```python
from build123d import *

# Parameters (mm, degrees)
SKETCH1_W               = 100
SKETCH1_H               = 100
BOSS_EXTRUDE1_DEPTH     = 20
SKETCH3_R               = 7.1
CUT_EXTRUDE1_DEPTH      = 16.5
CUT_EXTRUDE4_DEPTH      = 74.484692283
CUT_EXTRUDE4_DEPTH_BACK = 74.484692283
SKETCH7_R               = 6.1
FILLET1_R               = 3
SKETCH11_W              = 24
SKETCH11_H              = 24
CUT_EXTRUDE6_DEPTH      = 15
SKETCH12_W              = 18
SKETCH12_H              = 15
CUT_EXTRUDE7_DEPTH      = 32


with BuildPart() as part:
    # Sketch1 → Boss-Extrude1 (new body)
    with BuildSketch(Plane(origin=(0, 0, 0), x_dir=(1, 0, 0), z_dir=(0, 1, 0))):
        Rectangle(SKETCH1_W, SKETCH1_H)
    extrude(amount=BOSS_EXTRUDE1_DEPTH)

    # Sketch3 → Cut-Extrude1 (cut)
    with BuildSketch(Plane(origin=(0, 20, 0), x_dir=(1, 0, 0), z_dir=(0, 1, 0))):
        with Locations(Location((0, 0, 0), (0, 0, 270))):
            Circle(SKETCH3_R)
    extrude(amount=-CUT_EXTRUDE1_DEPTH, mode=Mode.SUBTRACT)

    # Sketch7 → Cut-Extrude4 (cut, two sides: drawn at the far end of the back side and taken through both)
    with BuildSketch(Plane(origin=(0, 0, 0), x_dir=(0, 0, -1), z_dir=(1, 0, 0)).offset(-CUT_EXTRUDE4_DEPTH_BACK)):
        with Locations((30, 12.5)):
            Circle(SKETCH7_R)
        with Locations(Location((-30, 12.5, 0), (0, 0, 180))):
            Circle(SKETCH7_R)
    extrude(amount=CUT_EXTRUDE4_DEPTH + CUT_EXTRUDE4_DEPTH_BACK, mode=Mode.SUBTRACT)

    # Fillet1
    fillet1_edges = [part.edges().sort_by_distance(p)[0] for p in [
        (50, 10, 50),
        (-50, 10, 50),
        (-50, 10, -50),
        (50, 10, -50),
    ]]
    fillet(fillet1_edges, radius=FILLET1_R)

    # Sketch11 → Cut-Extrude6 (cut)
    with BuildSketch(Plane(origin=(0, 20, 0), x_dir=(1, 0, 0), z_dir=(0, 1, 0))):
        Polygon((-50, 12), (-28, 12), (-28, 50), (28, 50), (28, 12), (50, 12), (50, -12), (28, -12), (28, -50), (-28, -50), (-28, -12), (-50, -12), align=None)
        Rectangle(SKETCH11_W, SKETCH11_H, mode=Mode.SUBTRACT)
    extrude(amount=-CUT_EXTRUDE6_DEPTH, mode=Mode.SUBTRACT)

    # Sketch12 → Cut-Extrude7 (cut)
    with BuildSketch(Plane(origin=(12, 0, 0), x_dir=(0, 0, -1), z_dir=(1, 0, 0))):
        with Locations((0, 12.5)):
            Rectangle(SKETCH12_W, SKETCH12_H)
    extrude(amount=-CUT_EXTRUDE7_DEPTH, mode=Mode.SUBTRACT)


solid = part.part
```
The listing builds one solid part. Answer for the finished solid, in the listing's coordinates (mm). A direction names the side the tool comes from. Round coordinates to 2 decimals unless told otherwise and drop trailing zeros. Write each loop counter-clockwise with the first axis right and the second up, starting at its lowest first coordinate (ties: lowest second). Pieces come first, ordered by that corner, then holes. Notation, with made-up numbers: (-40, -21.5) -> (-19, -21.5) arc R27 cw to (-19, 7.5) -> close; hole circle Ø4 at (63, 57). An arc over 180 degrees is marked (long way). Use CSV: the item, a comma, the result in double quotes. Start each with the question number.
(1) Section B-B on x = -29.5 is taken. Give the vertices of the cut face in (y, z).
(2) Which of the six approach directions +Z, -Z, +X, -X, +Y, -Y give full straight-line access (tool end or side, diameter ignored) to faces 1 (the face through (0, 12, 9)), 2 (the face through (12, 13, -10)), 3 (the face through (-12, 13, -10))?
(3) Section A-A on z = -30 is taken. Give the vertices of the cut face in (x, y), then the cut area to 3 significant figures.
(4) Consider L1, parallel to X at y = 4.5, z = 0; L2, parallel to Y at x = 36.5, z = -30; L3, parallel to Y at x = 6, z = -25.5. Determine where each line is inside the solid, lowest interval first. Write a range as from..to.
(5) Section C-C on z = 0 is taken. Give the vertices of the cut face in (x, y).
(6) The mould has two halves that part along Y. Classify faces 4 (the face through (-39.154, 7.088, -32.815)), 5 (the face through (39, 20, 31)), 6 (the face through (-12, 13, 11)), 7 (the face through (38.846, 7.088, -32.815)): released by +Y, released by -Y, zero draft, split by the parting line, or undercut.
(7) Section D-D on y = 12.5 is taken. Count the separate pieces of the cut face and the enclosed holes in it, then the cut area to 3 significant figures.
(8) Each of these flat-tipped pins is pushed along its axis until it touches: pin 1 (12 mm diameter, centred on x = -2.5, y = 16, fed in from -Z); pin 2 (3.5 mm diameter, centred on y = 14, z = -11, fed in from +X); pin 3 (11.5 mm diameter, centred on x = 0, z = 0, fed in from +Y); pin 4 (2.5 mm diameter, centred on y = 11, z = 10.5, fed in from +X). Where does it stop, or does it pass through?
A:
1,outline,"(0, -50) -> (20, -50) -> (20, -12) -> (5, -12) -> (5, 12) -> (20, 12) -> (20, 50) -> (0, 50) -> close; hole circle Ø12.2 at (12.5, -30); hole circle Ø12.2 at (12.5, 30)"
2,face 1,"+X, -X, +Y"
2,face 2,"+Z, -Z, +X, +Y"
2,face 3,"+Z, -Z, -X, +Y"
3,outline,"(-50, 0) -> (50, 0) -> (50, 6.4) -> (28, 6.4) -> (28, 5) -> (-28, 5) -> (-28, 6.4) -> (-50, 6.4) -> close; (-50, 18.6) -> (-28, 18.6) -> (-28, 20) -> (-50, 20) -> close; (28, 18.6) -> (50, 18.6) -> (50, 20) -> (28, 20) -> close"
3,area,"623 mm²"
4,L1,"x = -50..-7.1, 7.1..50"
4,L2,"y = 0..6.4, 18.6..20"
4,L3,"y = 0..5"
5,outline,"(-50, 0) -> (50, 0) -> (50, 5) -> (7.1, 5) -> (7.1, 3.5) -> (-7.1, 3.5) -> (-7.1, 5) -> (-50, 5) -> close"
6,face 4,"undercut"
6,face 5,"released by +Y"
6,face 6,"zero draft"
6,face 7,"undercut"
7,separate pieces,"10"
7,enclosed holes,"0"
7,area,"2,410 mm²"
8,pin 1,"stops at z = -12"
8,pin 2,"stops at x = 50"
8,pin 3,"stops at y = 3.5"
8,pin 4,"stops at x = 12"
